Autodesk Fusion 360 part; units mm, degrees
sketch "Sketch1" plane through (0, 0, 0) normal (0, 1, 0) x (1, 0, 0)
  line L0 (0, 0) -> (4.95, 0) construction
  line L1 (4.95, 0) -> (5.5, 0)
  line L2 (5.5, 0) -> (5.5, -0.63)
  line L3 (4.95, 0) -> (4.95, -2.5)
  line L4 (5.5, -0.63) -> (7.95, -0.63)
  line L5 (0, 0) -> (0, -2.6) construction
  line L6 (4.95, -2.5) -> (5.5, -2.5)
  line L7 (5.5, -2.5) -> (5.5, -2.4)
  line L8 (5.5, -2.4) -> (6.5, -2.4)
  line L9 (7.95, -0.63) -> (7.95, -1.13)
  line L10 (6.5, -2.4) -> (7.95, -1.13)
  dimension "d1" = 4.95
  dimension "d2" = 0.55
  dimension "d3" = 0.63
  dimension "d6" = 3
  dimension "d7" = 0.55
  dimension "d8" = 0.1
  dimension "d9" = 1.55
  dimension "d10" = 0.5
  dimension "d11" = 2.5
revolve "Revolve1" add sketch "Sketch1" angle 360 about axis through (0, 0, 0) along (0, 0, 1)
equation "d1 = ( 9.9 / 2 ) * 1 mm"
Here's how the part is built. I have some questions about the finished solid (model axes, mm). Coordinates: 2 decimals unless noted, no trailing zeros. Loops run counter-clockwise (first coordinate to the right, second up) from the corner with the lowest first, then second, coordinate; pieces in that order, holes last.
1. I need wall thicknesses on L1, parallel to Y at x = 0, z = 1; L2, parallel to Z at x = -0.75, y = -6.25; L3, parallel to X at y = 0.75, z = 1.65. Which ranges of each line are inside material? Lowest first, please.
2. If we mould it in two halves opening along Y, with no side actions, what happens to faces 1 (the flat face through (-5, 3, 2.4)), 2 (the cylindrical face through (-1.72, -7.76, 0.88)), 3 (the cylindrical face through (4.72, 1.49, 1.27))? For each: pulls with the +Y half, pulls with the -Y half, needs draft (parallel to the pull), parting line crosses it, or undercut.
3. Imagine slicing it at A-A, the plane x = 0. Please give me the cut outline in (y, z).
4. For P1, Ø1.5, axis at y = -1.5, z = 1.5, coming from the +X side; P2, Ø1, axis at x = -0.5, z = 1.5, coming from the +Y side, each with a flat end and sliding along its axis, tell me the tip position at first contact or that it passes through.
5. Imagine slicing it at C-C, the plane z = 1.5. Please give me the cut outline in (x, y), and give its area (3 significant figures).
Taken from the geometry:
1. L1: y = -7.95 to -4.95, 4.95 to 7.95
1. L2: z = 0.63 to 2.4
1. L3: x = -7.32 to -4.89, 4.89 to 7.32
2. face 1: needs draft
2. face 2: parting line crosses it
2. face 3: undercut
3. outline: (-7.95, 0.63) - (-5.5, 0.63) - (-5.5, 0) - (-4.95, 0) - (-4.95, 2.5) - (-5.5, 2.5) - (-5.5, 2.4) - (-6.5, 2.4) - (-7.95, 1.13) - close; (4.95, 0) - (5.5, 0) - (5.5, 0.63) - (7.95, 0.63) - (7.95, 1.13) - (6.5, 2.4) - (5.5, 2.4) - (5.5, 2.5) - (4.95, 2.5) - close
4. P1: stops at x = 7.9
4. P2: stops at y = 7.95
5. outline: circle Ø15.06 at (0, 0); hole circle Ø9.9 at (0, 0)
5. area: 101 mm2
